The model under review builds one solid part; all positions refer to its coordinate system, in mm. A direction names the side the tool comes from. Give positions to 0.01 mm unless a question says otherwise; leave off trailing zeros. Order: outer loops, then holes, each group sorted by start corner. A loop starts at its lowest first (then second) coordinate and runs counter-clockwise, first axis right, second up. Notation, with made-up numbers: M 61.25,6.25 L 87.25,6.25 A14 ccw 87.25,18.25 Z; hole C 46.25,35 d3. An arc over 180 degrees is marked long. One line per question, with ' | ' between items. Start each with the question number.
1. The part is to be moulded in two halves that separate along X. For faces 1 (the face through (3, -6, -34)), 2 (the face through (0, -4, -34)), 3 (the face through (116, -4, -34)), say which applies: +X half, -X half, draft (parallel to the pull), parting line (faces both ways), or undercut.
2. We need section B-B on z = -48. Write out the cut boundary in (x, y).
3. We need section C-C on y = 3.5. Write out the cut boundary in (x, z).
4. We need section D-D on x = 106. Write out the cut boundary in (y, z).
5. Wall thickness on L1, parallel to X at y = 2.75, z = -42; L2, parallel to X at y = -10.25, z = -9; L3, parallel to Z at x = 61, y = -8.75: over which ranges is each line inside the solid? List them lowest first.
6. For faces 4 (the face through (57, -6, -64)), 5 (the face through (57, -4, 0)), 6 (the face through (69, 2, -45.18)), list the 3-axis set-ups (+Z, -Z, +X, -X, +Y, -Y) from which the entire face can be reached by the end or side of a thin tool; tool diameter is ignored.
7. We need section A-A on z = -38. Write out the cut boundary in (x, y).
```python
from build123d import *

# Parameters (mm, degrees)
SKETCH1_W           = 116
SKETCH1_H           = 67
BOSS_EXTRUDE1_DEPTH = 5
SKETCH2_W           = 116
SKETCH2_H           = 67
SKETCH2_W_2         = 110
SKETCH2_H_2         = 61
BOSS_EXTRUDE2_DEPTH = 12.35
SKETCH3_W           = 28
SKETCH3_H           = 35.6
CUT_EXTRUDE1_DEPTH  = 135.527032599
SKETCH4_W           = 10
SKETCH4_H           = 10
CUT_EXTRUDE2_DEPTH  = 135.527032599
SKETCH5_W           = 5
SKETCH5_H           = 12
CUT_EXTRUDE3_DEPTH  = 135.527032599


with BuildPart() as part:
    # Sketch1 → Boss-Extrude1 (new body)
    with BuildSketch(Plane(origin=(0, 0, 0), x_dir=(1, 0, 0), z_dir=(0, 1, 0))):
        with Locations((58, 33.5)):
            Rectangle(SKETCH1_W, SKETCH1_H)
    extrude(amount=BOSS_EXTRUDE1_DEPTH)

    # Sketch2 → Boss-Extrude2 (add)
    with BuildSketch(Plane.XZ):
        with Locations((58, -33.5)):
            Rectangle(SKETCH2_W, SKETCH2_H)
        with Locations((58, -33.5)):
            Rectangle(SKETCH2_W_2, SKETCH2_H_2, mode=Mode.SUBTRACT)
    extrude(amount=BOSS_EXTRUDE2_DEPTH)

    # Sketch3 → Cut-Extrude1 (cut, through all)
    with BuildSketch(Plane.XZ):
        with Locations((95.8, -43.2)):
            Rectangle(SKETCH3_W, SKETCH3_H)
    extrude(amount=-CUT_EXTRUDE1_DEPTH, mode=Mode.SUBTRACT)

    # Sketch4 → Cut-Extrude2 (cut, through all)
    with BuildSketch(Plane.XZ):
        with Locations((68.7, -40.18)):
            Rectangle(SKETCH4_W, SKETCH4_H)
    extrude(amount=-CUT_EXTRUDE2_DEPTH, mode=Mode.SUBTRACT)

    # Sketch5 → Cut-Extrude3 (cut, through all)
    with BuildSketch(Plane.XZ):
        with Locations((11.8, -19.05)):
            Rectangle(SKETCH5_W, SKETCH5_H)
    extrude(amount=-CUT_EXTRUDE3_DEPTH, mode=Mode.SUBTRACT)


solid = part.part
```
Entries:
1) face 1: undercut | face 2: -X half | face 3: +X half
2) outline: M 0,-12.35 L 3,-12.35 L 3,0 L 81.8,0 L 81.8,5 L 0,5 Z; M 109.8,0 L 113,0 L 113,-12.35 L 116,-12.35 L 116,5 L 109.8,5 Z
3) outline: M 0,-67 L 116,-67 L 116,0 L 0,0 Z; hole M 9.3,-25.05 L 14.3,-25.05 L 14.3,-13.05 L 9.3,-13.05 Z; hole M 63.7,-45.18 L 73.7,-45.18 L 73.7,-35.18 L 63.7,-35.18 Z; hole M 81.8,-61 L 109.8,-61 L 109.8,-25.4 L 81.8,-25.4 Z
4) outline: M -12.35,-67 L 5,-67 L 5,-61 L 0,-61 L 0,-64 L -12.35,-64 Z; M -12.35,-3 L 0,-3 L 0,-25.4 L 5,-25.4 L 5,0 L -12.35,0 Z
5) L1: x = 0 to 63.7, 73.7 to 81.8, 109.8 to 116 | L2: x = 0 to 3, 113 to 116 | L3: z = -67 to -64, -3 to 0
6) face 4: -Y | face 5: +Z, +X, -X, +Y, -Y | face 6: +Y, -Y
7) outline: M 0,-12.35 L 3,-12.35 L 3,0 L 63.7,0 L 63.7,5 L 0,5 Z; M 73.7,0 L 81.8,0 L 81.8,5 L 73.7,5 Z; M 109.8,0 L 113,0 L 113,-12.35 L 116,-12.35 L 116,5 L 109.8,5 Z
